Source: CAD feature listing. Evaluate the final solid. Frame: model axes, mm. A direction names the side the tool comes from. Give positions to 0.01 mm unless a question says otherwise; leave off trailing zeros. Write each loop counter-clockwise with the first axis right and the second up, starting at its lowest first coordinate (ties: lowest second). Pieces come first, ordered by that corner, then holes. Notation, with made-up numbers: M 32.5,-18 L 71.5,-18 A20 ccw 71.5,6 Z; hole C -11,78.5 d3. An arc over 180 degrees is marked long. Return JSON: item names as keys, results as strings.
```python
from build123d import *

# Parameters (mm, degrees)
F0_W     = 190.5
F0_H     = 127
F1_DEPTH = 12.7
F2_W     = 3.175
F2_H     = 50.8
F3_DEPTH = 25.4
F4_W     = 3.175
F4_H     = 50.8
F5_DEPTH = 25.4
F7_D     = 3.175


with BuildPart() as f1:
    # F0 (on Front) → F1 (new body)
    with BuildSketch(Plane.XZ):
        Polygon((0, 571.5), (0, 0), (215.9, 0), (215.9, 571.5), (203.2, 571.5), (12.7, 571.5), align=None)
        with Locations((107.95, 76.2)):
            Rectangle(F0_W, F0_H, mode=Mode.SUBTRACT)
        with Locations((107.95, 215.9)):
            Rectangle(F0_W, F0_H, mode=Mode.SUBTRACT)
        with Locations((107.95, 355.6)):
            Rectangle(F0_W, F0_H, mode=Mode.SUBTRACT)
        with Locations((107.95, 495.3)):
            Rectangle(F0_W, F0_H, mode=Mode.SUBTRACT)
    extrude(amount=F1_DEPTH)

    # F2 (on face) → F3 (join)
    with BuildSketch(Plane.XZ.offset(12.7)):
        with Locations((214.3125, 495.3)):
            Rectangle(F2_W, F2_H)
    extrude(amount=F3_DEPTH)

    # F4 (on face) → F5 (join)
    with BuildSketch(Plane.XZ.offset(12.7)):
        with Locations((214.3125, 76.2)):
            Rectangle(F4_W, F4_H)
    extrude(amount=F5_DEPTH)

    # F7 (through all)
    with Locations(Plane(origin=(212.725, 0, 0), x_dir=(0, -1, 0), z_dir=(-1, 0, 0))):
        with Locations((25.4, 495.3), (25.4, 76.2)):
            Hole(F7_D / 2)


solid = f1.part
```
1) Cut plane B-B, the plane y = -5. Return the cut outline in (x, z), then the cut area to 3 significant figures.
Numbers:
{"outline": "M 0,0 L 215.9,0 L 215.9,571.5 L 0,571.5 Z; hole M 12.7,12.7 L 203.2,12.7 L 203.2,139.7 L 12.7,139.7 Z; hole M 12.7,152.4 L 203.2,152.4 L 203.2,279.4 L 12.7,279.4 Z; hole M 12.7,292.1 L 203.2,292.1 L 203.2,419.1 L 12.7,419.1 Z; hole M 12.7,431.8 L 203.2,431.8 L 203.2,558.8 L 12.7,558.8 Z", "area": "26,600 mm²"}
2) Cut plane D-D, the plane y = -32.5. Return the cut outline in (x, z) (3 decimals), then the cut area to 3 significant figures.
Numbers:
{"outline": "M 212.725,50.8 L 215.9,50.8 L 215.9,101.6 L 212.725,101.6 Z; M 212.725,469.9 L 215.9,469.9 L 215.9,520.7 L 212.725,520.7 Z", "area": "323 mm²"}
3) Cut plane A-A, the plane z = 511. Return the cut outline in (x, y) (3 decimals), then the cut area to 3 significant figures.
Numbers:
{"outline": "M 0,-12.7 L 12.7,-12.7 L 12.7,0 L 0,0 Z; M 203.2,-12.7 L 212.725,-12.7 L 212.725,-38.1 L 215.9,-38.1 L 215.9,0 L 203.2,0 Z", "area": "403 mm²"}
4) Contact query for flat-ended pins moving along their axis: pin 1 Ø1 at (x, y) = (214, -28) entering from +Z; pin 2 Ø7.5 at (y, z) = (-31.5, 66) entering from -X (3 decimals); pin 3 Ø1 at (x, y) = (214, -19.5) entering from -Z. Output: stop coordinate, or through.
Numbers:
{"pin 1": "stops at z = 520.7", "pin 2": "stops at x = 212.725", "pin 3": "stops at z = 50.8"}
5) Draft query along Z for faces 3 (the face through (0, -6, 290)), 4 (the face through (106, -6, 0)), 5 (the face through (203.2, -6, 215)), 6 (the face through (109, -6, 571.5)). Return one class per face: released by +Z, released by -Z, zero draft, split by the parting line, or undercut.
Numbers:
{"face 3": "zero draft", "face 4": "released by -Z", "face 5": "undercut", "face 6": "released by +Z"}
6) Cut plane C-C, the plane x = 45. Return the cut outline in (y, z), then the cut area to 3 significant figures.
Numbers:
{"outline": "M -12.7,0 L 0,0 L 0,12.7 L -12.7,12.7 Z; M -12.7,139.7 L 0,139.7 L 0,152.4 L -12.7,152.4 Z; M -12.7,279.4 L 0,279.4 L 0,292.1 L -12.7,292.1 Z; M -12.7,419.1 L 0,419.1 L 0,431.8 L -12.7,431.8 Z; M -12.7,558.8 L 0,558.8 L 0,571.5 L -12.7,571.5 Z", "area": "806 mm²"}
7) Set-up query: faces 1 (the face through (215.9, -10, 282)), 2 (the face through (12.7, -6, 75)). Return all of +Z, -Z, +X, -X, +Y, -Y with unobstructed straight access to the full face (end or side cutting, diameter ignored); none if empty.
Numbers:
{"face 1": "+Z, -Z, +X, +Y, -Y", "face 2": "+Y, -Y"}
8) Line query: line 1 (Z direction, x = 42.5, y = -6.5); line 2 (Z direction, x = 213.5, y = -25.4); line 3 (X direction, y = -11, z = 210.5). Output: solid intervals per line, ascending. Write a range as [from, to].
Numbers:
{"line 1": "z = [0, 12.7], [139.7, 152.4], [279.4, 292.1], [419.1, 431.8], [558.8, 571.5]", "line 2": "z = [50.8, 74.61], [77.79, 101.6], [469.9, 493.71], [496.89, 520.7]", "line 3": "x = [0, 12.7], [203.2, 215.9]"}
